Autodesk Inventor part; units mm, degrees
ref_plane "Work Plane1" through (0, 0, 86) normal (0, 0, 1) x (1, 0, 0)
ref_plane "YZ Plane" through (0, 0, 0) normal (1, 0, 0) x (0, 1, 0)
ref_plane "XZ Plane" through (0, 0, 0) normal (0, 1, 0) x (-1, 0, 0)
sketch "Sketch1" plane through (0, 0, 0) normal (0, 0, 1) x (1, 0, 0)
  line L0 (0, -21) -> (0, 21)
  line L1 (0, 15) -> (0, -15)
  line L2 (0, -15) -> (-0.4, -15)
  line L3 (-0.4, -15) -> (-15, 0)
  line L4 (-15, 0) -> (-0.4, 15)
  line L5 (-0.4, 15) -> (0, 15)
  point P0 (0, 0)
  point P1 (0, 0)
  dimension "d1" = 30
  dimension "d5" = 15
  dimension "d50" = 0.4
  dimension "d51" = 15
ref_plane "Work Plane1" through (0, 0, 86) normal (0, 0, 1) x (1, 0, 0)
sketch "Sketch2" plane through (0, 0, 86) normal (0, 0, 1) x (1, 0, 0)
  line L0 (0, -21) -> (0, 21)
  line L1 (0, 15) -> (0, -15)
  line L2 (0, -15) -> (-0.4, -15)
  line L3 (-0.4, -15) -> (-6, 0)
  line L4 (-6, 0) -> (-0.4, 15)
  line L5 (-0.4, 15) -> (0, 15)
  point P0 (0, 0)
  dimension "d3" = 30
  dimension "d6" = 15
  dimension "d52" = 0.4
  dimension "d53" = 6
loft "Loft1" add profiles "Sketch2", "Sketch1"
sketch "Sketch3" plane through (0, -15, 86) normal (1, 0, 0) x (0, 0, -1)
  line L0 (0, 30) -> (86, 30)
  line L1 (0, 0) -> (86, 0)
  line L2 (0, 30) -> (6, 30)
  line L3 (6, 30) -> (6, 0)
  line L4 (6, 0) -> (0, 0)
  line L5 (0, 0) -> (0, 30)
  line L6 (74, 30) -> (80, 30)
  line L7 (80, 30) -> (80, 0)
  line L8 (80, 0) -> (74, 0)
  line L9 (74, 0) -> (74, 30)
  point P0 (86, 15)
  point P1 (74, 0)
  dimension "d11" = 6
  dimension "d12" = 6
  dimension "d13" = 6
extrude "Extrusion1" add sketch "Sketch3" along normal blind 16.51 contours L0 L3 L1 L5 | L0 L7 L1 L9
sketch "Sketch4" plane through (0, -15, 80) normal (1, 0, 0) x (0, 0, -1)
  circle A0 centre (37.25, 15) radius 1.75
  line L0 (-6, 30) -> (-6, 0)
  line L1 (-6, 15) -> (80, 15)
  dimension "d16" = 43.25
  dimension "d17" = 3.5
extrude "Extrusion2" cut sketch "Sketch4" against normal through all
sketch "Sketch5" plane through (0, -15, 0) normal (0, 0, -1) x (-1, 0, 0)
  line L0 (0, 0) -> (0, 30)
  circle A0 centre (6.2132, 15) radius 6.2132
  line L1 (15, 15) -> (0, 0)
  line L2 (0, 30) -> (15, 15)
  line L3 (0, 0) -> (0, 30)
  circle A1 centre (6.2132, 15) radius 1.75
  line L4 (0.4, 30) -> (15, 15)
  line L5 (0, 30) -> (0.4, 30)
  line L6 (0.4, 0) -> (0, 0)
  line L7 (15, 15) -> (0.4, 0)
  point P0 (0, 15)
  dimension "d20" = 3.5
extrude "Extrusion3" add sketch "Sketch5" along normal blind 3 contours A1
sketch "Sketch6" plane through (16.51, -15, 86) normal (1, 0, 0) x (0, 0, -1)
  line L0 (6, 0) -> (6, 30)
  line L1 (6, 30) -> (0, 30)
  line L2 (0, 30) -> (0, 0)
  line L3 (0, 0) -> (6, 0)
  point P0 (86, 15)
extrude "Extrusion4" add sketch "Sketch6" along normal blind 12
sketch "Sketch8" plane through (16.51, -15, 86) normal (1, 0, 0) x (0, 0, -1)
  line L0 (74, 3) -> (80, 3)
  line L1 (74, 0) -> (80, 0)
  line L2 (74, 27) -> (80, 27)
  line L3 (80, 30) -> (74, 30)
  line L4 (74, 0) -> (74, 30)
  line L5 (74, 21) -> (80, 21)
  line L6 (74, 9) -> (80, 9)
  circle A0 centre (77, 21) radius 1.45
  circle A1 centre (77, 9) radius 1.45
  line L7 (80, 0) -> (80, 30)
  point P0 (86, 15)
  dimension "d25" = 3
  dimension "d26" = 3
  dimension "d27" = 6
  dimension "d28" = 6
  dimension "d29" = 2.9
  dimension "d30" = 2.9
  dimension "d48" = 3
  dimension "d49" = 3
extrude "Extrusion5" cut sketch "Sketch8" against normal blind 7 contours A1 L6 | L6 A1 | A0 L5 | L5 A0
sketch "Sketch9" plane through (0, -15, 86) normal (0, 0, 1) x (1, 0, 0)
  line L0 (0, 30) -> (28.51, 30)
  line L1 (22.51, 30) -> (22.51, 0.0044)
  line L2 (28.51, 30) -> (28.51, 0)
  line L3 (28.51, 30) -> (0, 30)
  line L4 (-0.4, 0) -> (28.51, 0)
  line L5 (28.51, 3) -> (0.1043, 3)
  line L6 (28.51, 27) -> (0.4735, 27)
  line L7 (25.51, 30) -> (25.51, 0)
  line L8 (22.51, 21) -> (28.51, 21)
  line L9 (28.51, 0) -> (28.51, 30)
  line L10 (22.51, 9) -> (28.51, 9)
  circle A0 centre (25.51, 21) radius 1.45
  circle A1 centre (25.51, 9) radius 1.45
  point P0 (0, 15)
  point P1 (16.51, 0)
  point P2 (16.51, 30)
  point P3 (0, 0)
  dimension "d33" = 6
  dimension "d35" = 3
  dimension "d36" = 3
  dimension "d43" = 3
  dimension "d44" = 6
  dimension "d45" = 6
  dimension "d46" = 2.9
  dimension "d47" = 2.9
extrude "Extrusion6" cut sketch "Sketch9" against normal up to surface (6 mm away) contours A0 L8 L7 | L7 L8 A0 | L8 L7 A0 | L8 A0 L7 | A1 L7 L10 | L10 L7 A1 | L10 A1 L7 | L7 A1 L10
sketch "Sketch10" plane through (28.51, -15, 86) normal (1, 0, 0) x (0, 0, -1)
  line L0 (6, 30) -> (0, 30)
  line L1 (0, 30) -> (0, 0)
  line L2 (0, 0) -> (6, 0)
  line L3 (6, 0) -> (6, 30)
  point P0 (86, 15)
extrude "Extrusion7" add sketch "Sketch10" along normal blind 3
equation "\"d1\" = Height"
equation "\"d51\" = SideArmorWidth"
equation "\"d3\" = Height"
equation "\"d53\" = SideThickness"
equation "\"d11\" = SideThickness"
equation "\"d12\" = SideThickness"
equation "\"d13\" = SideThickness"
equation "\"d14\" = WheelWidth"
equation "\"d16\" = DriveMotorOffset + SideThickness"
equation "\"d17\" = DriveMotorHoleDia"
equation "\"d20\" = ForkPlugDia"
equation "\"d21\" = ForkPlugLength"
equation "\"d23\" = 2 * SideThickness"
equation "\"d25\" = BaseThickness"
equation "\"d26\" = BaseThickness"
equation "\"d27\" = SideThickness"
equation "\"d28\" = SideThickness"
equation "\"d29\" = ScrewDia"
equation "\"d30\" = ScrewDia"
equation "\"d48\" = 0.5 * SideThickness"
equation "\"d49\" = 0.5 * SideThickness"
equation "\"d31\" = ScrewDepth"
equation "\"d33\" = SideThickness"
equation "\"d35\" = BaseThickness"
equation "\"d36\" = BaseThickness"
equation "\"d43\" = 0.5 * SideThickness"
equation "\"d44\" = SideThickness"
equation "\"d45\" = SideThickness"
equation "\"d46\" = ScrewDia"
equation "\"d47\" = ScrewDia"
equation "\"d2\" = BoxLength + SideThickness"
properties part number "BodyWedgeSideV3.1" material "Thermoplastic Resin"
Geometry: final body of the model. Coordinates: model frame, mm. A direction names the side the tool comes from. Give positions to 0.01 mm unless a question says otherwise; leave off trailing zeros. Order: outer loops, then holes, each group sorted by start corner. A loop starts at its lowest first (then second) coordinate and runs counter-clockwise, first axis right, second up. Notation, with made-up numbers: (76.5, 86.5) -> (118.5, 86.5) arc R27 cw to (118.5, 120.5) -> close; hole circle Ø9 at (32, 44). An arc over 180 degrees is marked (long way). Answer as a JSON object with one key per item and string values.
Q1. Draft query along Y for faces 1 (the flat face through (13, -15, 81)), 2 (the cylindrical face through (-7.83, 0.67, -1.48)), 3 (the cylindrical face through (26.89, 6.44, 83.04)), 4 (the flat face through (31.51, 0, 83)). Return one class per face: released by +Y, released by -Y, zero draft, split by the parting line, or undercut.
Entries:
{"face 1": "released by -Y", "face 2": "split by the parting line", "face 3": "undercut", "face 4": "zero draft"}
Q2. Section A-A (x = 25.51). Output: boundary loops of the cut face in (y, z).
Entries:
{"outline": "(-15, 80) -> (-7.45, 80) -> (-7.45, 86) -> (-15, 86) -> close; (-4.55, 80) -> (4.55, 80) -> (4.55, 86) -> (-4.55, 86) -> close; (7.45, 80) -> (15, 80) -> (15, 86) -> (7.45, 86) -> close"}
Q3. Section C-C (x = 19). Output: boundary loops of the cut face in (y, z), plus the area to 3 significant figures.
Entries:
{"outline": "(-15, 80) -> (15, 80) -> (15, 86) -> (-15, 86) -> close", "area": "180 mm^2"}
Q4. Section B-B (x = 4.5). Output: boundary loops of the cut face in (y, z).
Entries:
{"outline": "(-15, 6) -> (15, 6) -> (15, 12) -> (-15, 12) -> close; (-15, 80) -> (15, 80) -> (15, 86) -> (-15, 86) -> close"}
Q5. Access query for faces 5 (the flat face through (16, 0, 80)), 6 (the flat face through (16.51, 0, 9)), 7 (the cylindrical face through (13.06, -5.94, 10.45)), 8 (the flat face through (12, 0, 86)), 9 (the flat face through (13, 15, 81)). Directions: +Z, -Z, +X, -X, +Y, -Y. A direction counts if a zero-diameter tool reaches every point of the face in a straight line with its end or side. Return the directions, or none.
Entries:
{"face 5": "+X, +Y, -Y", "face 6": "-Z, +X, +Y, -Y", "face 7": "+X", "face 8": "+Z, +X, -X, +Y, -Y", "face 9": "+Z, -Z, +X, -X, +Y"}
Q6. First-contact query: pin 1 (1.8 mm diameter, centred on y = 1, z = 9.5, fed in from +X); pin 2 (2.5 mm diameter, centred on y = 6, z = 9, fed in from +X); pin 3 (12 mm diameter, centred on x = -2.5, y = -10, fed in from +Z); pin 4 (3 mm diameter, centred on y = 12, z = 54.5, fed in from +X). Flat tips, straight axial feed; report the tip coordinate or a pass-through.
Entries:
{"pin 1": "stops at x = 16.51", "pin 2": "stops at x = 9.51", "pin 3": "stops at z = 86", "pin 4": "stops at x = 0"}
Q7. Material intervals for probe 1 along Z at (x, y) = (13, -6); probe 2 along Y at (x, z) = (11.75, 9); probe 3 along Z at (x, y) = (9, -3), sorted ascending.
Entries:
{"probe 1": "z = 6 to 7.55, 10.45 to 12, 80 to 86", "probe 2": "y = -15 to -7.45, -4.55 to 4.55, 7.45 to 15", "probe 3": "z = 6 to 12, 80 to 86"}
